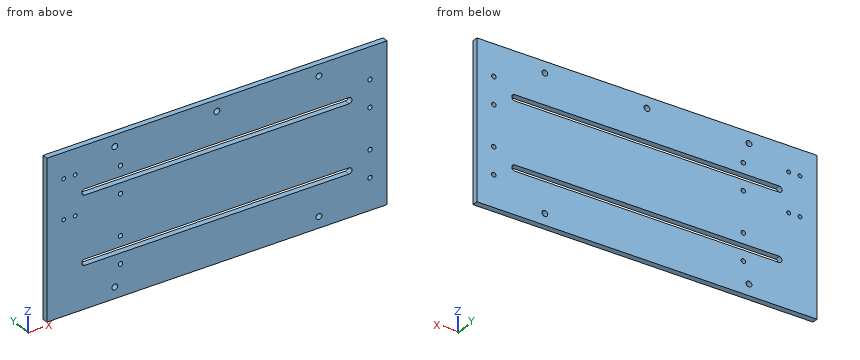
from build123d import *

# Parameters (mm, degrees)
SKETCH1_W                  = 381
SKETCH1_H                  = 177.8
PLATE_DEPTH                = 6.35
SKETCH4_R                  = 3.2639
CHASSISMOUNTINGHOLES_DEPTH = 6.35
SKETCH5_R                  = 2.5019
LEADSCREWGUIDEMOUNTS_DEPTH = 6.35
SKETCH6_R                  = 2.15265
LEADSCREWMOTORMOUNT_DEPTH  = 6.35
SKETCH8_R                  = 3.2639
CUT_EXTRUDE2_DEPTH         = 7.35
CUT_EXTRUDE4_DEPTH         = 7.35


with BuildPart() as part:
    # Sketch1 → Plate (new body)
    with BuildSketch(Plane(origin=(0, 0, 0), x_dir=(1, 0, 0), z_dir=(0, 1, 0))):
        Rectangle(SKETCH1_W, SKETCH1_H)
    extrude(amount=PLATE_DEPTH)

    # Sketch4 → ChassisMountingHoles (cut)
    with BuildSketch(Plane.XZ):
        with Locations((0, 76.2)):
            Circle(SKETCH4_R)
        with Locations((-114.3, 76.2)):
            Circle(SKETCH4_R)
        with Locations((114.3, 76.2)):
            Circle(SKETCH4_R)
        with Locations((-114.3, -76.2)):
            Circle(SKETCH4_R)
        with Locations((114.3, -76.2)):
            Circle(SKETCH4_R)
    extrude(amount=-CHASSISMOUNTINGHOLES_DEPTH, mode=Mode.SUBTRACT)

    # Sketch5 → LeadScrewGuideMounts (cut)
    with BuildSketch(Plane.XZ):
        with Locations((171.45, 53.34)):
            Circle(SKETCH5_R)
        with Locations((171.45, 22.86)):
            Circle(SKETCH5_R)
        with Locations((-107.95, 53.34)):
            Circle(SKETCH5_R)
        with Locations((-107.95, 22.86)):
            Circle(SKETCH5_R)
        with Locations((171.45, -53.34)):
            Circle(SKETCH5_R)
        with Locations((171.45, -22.86)):
            Circle(SKETCH5_R)
        with Locations((-107.95, -22.86)):
            Circle(SKETCH5_R)
        with Locations((-107.95, -53.34)):
            Circle(SKETCH5_R)
    extrude(amount=-LEADSCREWGUIDEMOUNTS_DEPTH, mode=Mode.SUBTRACT)

    # Sketch6 → LeadScrewMotorMount (cut)
    with BuildSketch(Plane.XZ):
        with Locations((-171.45, 60.325)):
            Circle(SKETCH6_R)
        with Locations((-158.75, 60.325)):
            Circle(SKETCH6_R)
        with Locations((-171.45, 15.875)):
            Circle(SKETCH6_R)
        with Locations((-158.75, 15.875)):
            Circle(SKETCH6_R)
    extrude(amount=-LEADSCREWMOTORMOUNT_DEPTH, mode=Mode.SUBTRACT)

    # Sketch8 → Cut-Extrude2 (cut, through all)
    with BuildSketch(Plane.XZ):
        with Locations((-25.4, 38.1)):
            Circle(SKETCH8_R)
        with Locations((25.4, 38.1)):
            Circle(SKETCH8_R)
        with Locations((76.2, 38.1)):
            Circle(SKETCH8_R)
    extrude(amount=-CUT_EXTRUDE2_DEPTH, mode=Mode.SUBTRACT)

    # Sketch10 → Cut-Extrude4 (cut, through all)
    with BuildSketch(Plane.XZ):
        with BuildLine():
            Line((-25.4, 41.4782), (-147.955, 41.4782))
            ThreePointArc((-147.955, 41.4782), (-151.3332, 38.1), (-147.955, 34.7218))
            Line((-147.955, 34.7218), (147.955, 34.7218))
            ThreePointArc((147.955, 34.7218), (151.3332, 38.1), (147.955, 41.4782))
            Line((147.955, 41.4782), (0, 41.4782))
            Line((0, 41.4782), (-25.4, 41.4782))
        make_face()
    cut_extrude4 = extrude(amount=-CUT_EXTRUDE4_DEPTH, mode=Mode.SUBTRACT)

    # Mirror3: Cut-Extrude4 across plane
    add(cut_extrude4.mirror(Plane.XY), mode=Mode.SUBTRACT)


solid = part.part
Here's how the part is built. I have some questions about the finished solid (model axes, mm). Round coordinates to 2 decimals unless told otherwise and drop trailing zeros. Write each loop counter-clockwise with the first axis right and the second up, starting at its lowest first coordinate (ties: lowest second). Pieces come first, ordered by that corner, then holes. Notation, with made-up numbers: (82.25, 81) -> (138.25, 81) arc R23 ccw to (138.25, 96) -> close; hole circle Ø5 at (62, 40). An arc over 180 degrees is marked (long way). One line per item, written item: value.
1) If I drill on line 1 (Z direction, x = -43.5, y = 1); line 2 (Z direction, x = 0, y = 4); line 3 (Z direction, x = -171, y = 6), over which ranges is the centre line in solid material (lowest first)? Write a range as [from, to].
Filled sheet:
line 1: z = [-88.9, -41.48], [-34.72, 34.72], [41.48, 88.9]
line 2: z = [-88.9, -41.48], [-34.72, 34.72], [41.48, 72.94], [79.46, 88.9]
line 3: z = [-88.9, 13.77], [17.98, 58.22], [62.43, 88.9]
2) I'm going to push a flat-ended pin straight in: pin 1 Ø4 at (x, z) = (114.3, -76.2) entering from +Y. Where does the tip first touch, or does it pass through?
Filled sheet:
pin 1: passes through
3) Suppose I cut it at B-B on y = 4.5. Give the number of separate pieces and of enclosed holes in the cut face, plus the area to 3 significant figures.
Filled sheet:
separate pieces: 1
enclosed holes: 19
area: 63,300 mm2
4) Suppose I cut it at A-A on x = -47. List the corners of the cut face in (y, z) for me, plus the area to 3 significant figures.
Filled sheet:
outline: (0, -88.9) -> (6.35, -88.9) -> (6.35, -41.48) -> (0, -41.48) -> close; (0, -34.72) -> (6.35, -34.72) -> (6.35, 34.72) -> (0, 34.72) -> close; (0, 41.48) -> (6.35, 41.48) -> (6.35, 88.9) -> (0, 88.9) -> close
area: 1,040 mm2
